Source: CAD feature listing. Evaluate the final solid. Frame: model axes, mm. A direction names the side the tool comes from. Coordinates: 2 decimals unless noted, no trailing zeros. Loops run counter-clockwise (first coordinate to the right, second up) from the corner with the lowest first, then second, coordinate; pieces in that order, holes last.
Item 1: Section query A-A, the plane z = 4.6. Return the cut outline in (x, y).
Item 2: Reachability of faces 4 (the flat face through (3, -0.5, -1)), 5 (the flat face through (-6.75, 0.5, -2)), 6 (the flat face through (-8.75, 0.2, 1.5)) from +Z, -Z, +X, -X, +Y, -Y: full face, straight path, thin tool, end or side. Return the list, or none.
Item 3: Pull-direction query (Z, two-part tool) for faces 1 (the cylindrical face through (3.8, -1, 7.1)), 2 (the flat face through (7, -1, 3)), 3 (the flat face through (2, 1, 0)); classes: +Z half, -Z half, draft (parallel to the pull), parting line (faces both ways), or undercut.
Item 4: Line query: probe 1 along X at (y, z) = (-1.3, 4.6); probe 2 along X at (y, z) = (0.5, 4.6); probe 3 along Y at (x, z) = (-0.75, 2.5). Output: solid intervals per line, ascending.
Item 5: Pin query (flat end, axial travel): pin 1 Ø6 at (x, z) = (-5.5, -4) entering from +Y; pin 2 Ø0.6 at (x, y) = (-3, -1.5) entering from -Z; pin 3 Ø1.6 at (x, z) = (3, 0) entering from -Y. Return the tip coordinate at first contact, or that it passes through.
Item 6: Section query D-D, the plane x = -0.75. Return the cut outline in (y, z).
Item 7: Section query C-C, the plane y = -1.8. Return the cut outline in (x, z).
Item 8: Section query B-B, the plane x = 7. Return the cut outline in (y, z), then the cut area to 3 significant figures.
```python
from build123d import *

# Parameters (mm, degrees)
CROQUIS1_R              = 1.5
SALIENTE_EXTRUIR1_DEPTH = 1
SALIENTE_EXTRUIR2_DEPTH = 2
CROQUIS3_W              = 2
CROQUIS3_H              = 6
SALIENTE_EXTRUIR3_DEPTH = 0.5


with BuildPart() as part:
    # Croquis1 → Saliente-Extruir1 (new body)
    with BuildSketch(Plane(origin=(0, 0, 0), x_dir=(1, 0, 0), z_dir=(0, 1, 0))):
        Polygon((-8.75, 7.25), (-6.75, 7.25), (0.75, 7.25), (8.75, 7.25), (8.75, -7.25), (-8.75, -7.25), align=None)
        with Locations(Location((3.75, -4.6, 0), (0, 0, 270))):
            Circle(CROQUIS1_R, mode=Mode.SUBTRACT)
        with BuildLine():
            Line((-6.75, 4.262531407), (-6.75, -0.237468593))
            ThreePointArc((-6.75, -0.237468593), (-3, -2.25), (0.75, -0.237468593))
            Line((0.75, -0.237468593), (0.75, 4.262531407))
            ThreePointArc((0.75, 4.262531407), (-3, 6.275062814), (-6.75, 4.262531407))
        make_face(mode=Mode.SUBTRACT)
    extrude(amount=SALIENTE_EXTRUIR1_DEPTH)

    # Croquis2 → Saliente-Extruir2 (add)
    with BuildSketch(Plane.XZ):
        with BuildLine():
            Line((-8.75, 7.25), (8.75, 7.25))
            Line((8.75, 7.25), (8.75, 3))
            Line((8.75, 3), (5.670937271, 3))
            ThreePointArc((5.670937271, 3), (3.75, 7.1), (1.829062729, 3))
            Line((1.829062729, 3), (-8.75, 3))
            Line((-8.75, 3), (-8.75, 7.25))
        make_face()
    extrude(amount=SALIENTE_EXTRUIR2_DEPTH)

    # Croquis3 → Saliente-Extruir3 (add)
    with BuildSketch(Plane.XZ):
        with Locations((2.75, -0.75)):
            Rectangle(CROQUIS3_W, CROQUIS3_H)
    extrude(amount=SALIENTE_EXTRUIR3_DEPTH)


solid = part.part
```
Verdict:
1. outline: (-8.75, -2) - (1.25, -2) - (1.25, 0) - (2.25, 0) - (2.25, 1) - (-8.75, 1) - close; (5.25, 0) - (6.25, 0) - (6.25, -2) - (8.75, -2) - (8.75, 1) - (5.25, 1) - close
2. face 4: -Z, +X, -X, -Y
2. face 5: +Y, -Y
2. face 6: +Z, -Z, -X, +Y, -Y
3. face 1: undercut
3. face 2: -Z half
3. face 3: draft
4. probe 1: x = -8.75 to 1.25, 6.25 to 8.75
4. probe 2: x = -8.75 to 2.25, 5.25 to 8.75
4. probe 3: y = 0 to 1
5. pin 1: stops at y = 1
5. pin 2: stops at z = 3
5. pin 3: stops at y = -0.5
6. outline: (-2, 3) - (0, 3) - (0, 1.65) - (1, 1.65) - (1, 7.25) - (-2, 7.25) - close; (0, -7.25) - (1, -7.25) - (1, -5.67) - (0, -5.67) - close
7. outline: (-8.75, 3) - (1.83, 3) arc R2.5 cw (long way) to (5.67, 3) - (8.75, 3) - (8.75, 7.25) - (-8.75, 7.25) - close
8. outline: (-2, 3) - (0, 3) - (0, -7.25) - (1, -7.25) - (1, 7.25) - (-2, 7.25) - close
8. area: 23.0 mm2
